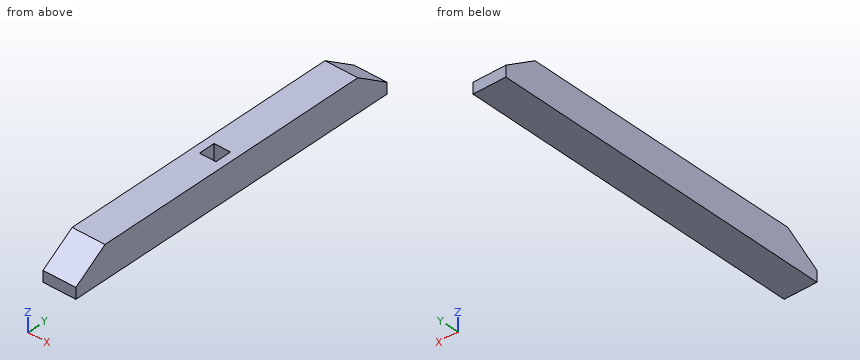
```python
from build123d import *

# Parameters (mm, degrees)
F1_DEPTH = 76.2
F2_W     = 38.1
F2_H     = 19.05
F3_DEPTH = 38.1


with BuildPart() as f1:
    # F0 (on Right) → F1 (new body)
    with BuildSketch(Plane.YZ):
        Polygon((406.4, -12.7), (330.2, 38.1), (-330.2, 38.1), (-406.4, -12.7), (-406.4, -38.1), (-292.1, -38.1), (292.1, -38.1), (406.4, -38.1), align=None)
    extrude(amount=F1_DEPTH)

    # F2 (on face) → F3 (cut)
    with BuildSketch(Plane.XY.offset(38.1)):
        with Locations((38.1, 9.525)):
            Rectangle(F2_W, F2_H)
        with Locations((38.1, -9.525)):
            Rectangle(F2_W, F2_H)
    extrude(amount=-F3_DEPTH, mode=Mode.SUBTRACT)


solid = f1.part
```
Build history of the part. All positions in model axes, mm. Round coordinates to 2 decimals unless told otherwise and drop trailing zeros. Write each loop counter-clockwise with the first axis right and the second up, starting at its lowest first coordinate (ties: lowest second). Pieces come first, ordered by that corner, then holes.
1) Pin check, flat tips, straight feed: pin 1 (6 mm diameter, centred on x = 12.5, z = -8, fed in from -Y); pin 2 (2 mm diameter, centred on y = -186.5, z = -28, fed in from -X); pin 3 (4 mm diameter, centred on x = 41, y = 17, fed in from +Z); pin 4 (5 mm diameter, centred on x = 41, z = -1, fed in from +Y). Stop position of each tip, or through.
2) Band-saw the part on A-A, the plane z = 23. List the corners of the cut face in (x, y).
3) Band-saw the part on B-B, the plane x = 12. List the corners of the cut face in (y, z).
4) Drill centre lines: probe 1 along Y at (x, z) = (42, 32); probe 2 along Y at (x, z) = (25, 21); probe 3 along Y at (x, z) = (63, 29). Where is each one in solid material? Low to high.
5) Band-saw the part on C-C, the plane x = 43. List the corners of the cut face in (y, z).
Ans:
1. pin 1: stops at y = -403.85
1. pin 2: stops at x = 0
1. pin 3: stops at z = 0
1. pin 4: stops at y = 392.6
2. outline: (0, -352.85) - (76.2, -352.85) - (76.2, 352.85) - (0, 352.85) - close; hole (19.05, -19.05) - (57.15, -19.05) - (57.15, 19.05) - (19.05, 19.05) - close
3. outline: (-406.4, -38.1) - (406.4, -38.1) - (406.4, -12.7) - (330.2, 38.1) - (-330.2, 38.1) - (-406.4, -12.7) - close
4. probe 1: y = -339.35 to -19.05, 19.05 to 339.35
4. probe 2: y = -355.85 to -19.05, 19.05 to 355.85
4. probe 3: y = -343.85 to 343.85
5. outline: (-406.4, -38.1) - (406.4, -38.1) - (406.4, -12.7) - (330.2, 38.1) - (19.05, 38.1) - (19.05, 0) - (-19.05, 0) - (-19.05, 38.1) - (-330.2, 38.1) - (-406.4, -12.7) - close
